Read the model definition and answer for the solid it produces. Units are mm, in the model's axes. A direction names the side the tool comes from. Round coordinates to 2 decimals unless told otherwise and drop trailing zeros. Write each loop counter-clockwise with the first axis right and the second up, starting at its lowest first coordinate (ties: lowest second). Pieces come first, ordered by that corner, then holes. Notation, with made-up numbers: (23.5, 77) - (55.5, 77) arc R26 ccw to (55.5, 100) - close; hole circle Ø9 at (69, -30). An arc over 180 degrees is marked (long way). One line per item, written item: value. Start each with the question number.
(1) The mould has two halves that part along Y. Classify faces 4 (the face through (77.33, -102.26, 774.52)), 5 (the face through (84.795, 26.703, 401.422)), 6 (the face through (127, 1, 775)): +Y half, -Y half, draft (parallel to the pull), parting line (faces both ways), or undercut.
(2) Flat-ended cylindrical pins translate along their axes: pin 1 Ø20.5 at (y, z) = (-34.5, 774) entering from -X; pin 2 Ø10 at (x, z) = (-37, 280.5) entering from +Y; pin 3 Ø12 at (x, z) = (10.5, 533.5) entering from +Y. Find the tip coordinate at first contact, or state that the pin passes through.
(3) A cutting plane is placed at D-D, the plane y = 64. Determine the outline of the cut face in (x, z), plus the area to 3 significant figures.
(4) A cutting plane is placed at A-A, the plane y = 0. Determine the outline of the cut face in (x, z).
(5) Find the intervals of material crossed by L1, parallel to X at y = -91, z = 771; L2, parallel to Y at x = 91.44, z = 769.5; L3, parallel to Y at x = 0, z = 305, in increasing order.
(6) A cutting plane is placed at C-C, the plane x = 0. Determine the outline of the cut face in (y, z).
(7) A cutting plane is placed at B-B, the plane x = -98. Determine the outline of the cut face in (y, z).
(8) For faces 1 (the face through (-110.86, -85.01, 25.04)), 2 (the face through (-73.677, -92.222, 774.522)), 3 (the face through (-2, -91, 50.8)), determine the directions among +Z, -Z, +X, -X, +Y, -Y from which every point of the face is accessible in a straight line to the end or side of a thin tool.
from build123d import *

# Parameters (mm, degrees)
SKETCH1_R           = 139.7
SKETCH1_R_2         = 88.9
BOSS_EXTRUDE3_DEPTH = 50.8
SKETCH1_4_R         = 88.9
SKETCH1_4_R_2       = 50.8
BOSS_EXTRUDE4_DEPTH = 762
SKETCH3_W           = 254
SKETCH3_H           = 247.65
SKETCH3_R           = 17.78
SKETCH3_R_2         = 50.8
BOSS_EXTRUDE5_DEPTH = 25.4


with BuildPart() as part:
    # Sketch1 → Boss-Extrude3 (new body)
    with BuildSketch(Plane.XY):
        Circle(SKETCH1_R)
        Circle(SKETCH1_R_2, mode=Mode.SUBTRACT)
    extrude(amount=BOSS_EXTRUDE3_DEPTH)

    # Sketch1_4 → Boss-Extrude4 (add)
    with BuildSketch(Plane.XY):
        Circle(SKETCH1_4_R)
        Circle(SKETCH1_4_R_2, mode=Mode.SUBTRACT)
    extrude(amount=BOSS_EXTRUDE4_DEPTH)

    # Sketch3 → Boss-Extrude5 (add)
    with BuildSketch(Plane.XY.offset(762)):
        with Locations((0, 3.175)):
            Rectangle(SKETCH3_W, SKETCH3_H)
        with Locations((-91.44, 91.44)):
            Circle(SKETCH3_R, mode=Mode.SUBTRACT)
        with Locations(Location((91.44, 91.44, 0), (0, 0, 180))):
            Circle(SKETCH3_R, mode=Mode.SUBTRACT)
        with Locations((91.44, -91.44)):
            Circle(SKETCH3_R, mode=Mode.SUBTRACT)
        with Locations(Location((-91.44, -91.44, 0), (0, 0, 180))):
            Circle(SKETCH3_R, mode=Mode.SUBTRACT)
        Circle(SKETCH3_R_2, mode=Mode.SUBTRACT)
    extrude(amount=BOSS_EXTRUDE5_DEPTH)


solid = part.part
Here are the results:
1. face 4: undercut
1. face 5: parting line
1. face 6: draft
2. pin 1: x = -127
2. pin 2: y = 82.94
2. pin 3: y = 88.79
3. outline: (-127, 762) - (-61.7, 762) - (-61.7, 50.8) - (-124.18, 50.8) - (-124.18, 0) - (124.18, 0) - (124.18, 50.8) - (61.7, 50.8) - (61.7, 762) - (127, 762) - (127, 787.4) - (-127, 787.4) - close
3. area: 107,000 mm²
4. outline: (-139.7, 0) - (-50.8, 0) - (-50.8, 787.4) - (-127, 787.4) - (-127, 762) - (-88.9, 762) - (-88.9, 50.8) - (-139.7, 50.8) - close; (50.8, 0) - (139.7, 0) - (139.7, 50.8) - (88.9, 50.8) - (88.9, 762) - (127, 762) - (127, 787.4) - (50.8, 787.4) - close
5. L1: -127 to -109.21, -73.67 to 73.67, 109.21 to 127
5. L2: -120.65 to -109.22, -73.66 to 73.66, 109.22 to 127
5. L3: -88.9 to -50.8, 50.8 to 88.9
6. outline: (-139.7, 0) - (-50.8, 0) - (-50.8, 787.4) - (-120.65, 787.4) - (-120.65, 762) - (-88.9, 762) - (-88.9, 50.8) - (-139.7, 50.8) - close; (50.8, 0) - (139.7, 0) - (139.7, 50.8) - (88.9, 50.8) - (88.9, 762) - (127, 762) - (127, 787.4) - (50.8, 787.4) - close
7. outline: (-120.65, 762) - (-107.97, 762) - (-107.97, 787.4) - (-120.65, 787.4) - close; (-99.56, 0) - (99.56, 0) - (99.56, 50.8) - (-99.56, 50.8) - close; (-74.91, 762) - (74.91, 762) - (74.91, 787.4) - (-74.91, 787.4) - close; (107.97, 762) - (127, 762) - (127, 787.4) - (107.97, 787.4) - close
8. face 1: -Z
8. face 2: +Z
8. face 3: none
